Geometry: final body of the model. Coordinates: model frame, mm. Round coordinates to 2 decimals unless told otherwise and drop trailing zeros. Loops run counter-clockwise (first coordinate to the right, second up) from the corner with the lowest first, then second, coordinate; pieces in that order, holes last. Notation, with made-up numbers: M 21,11.5 L 67,11.5 A16 ccw 67,26.5 Z; hole C 31.25,6 d5. An arc over 180 degrees is marked long. Return JSON: item names as keys, results as strings.
from build123d import *

# Parameters (mm, degrees)
SKETCH1_R                    = 42.5
BOSS_EXTRUDE1_DEPTH          = 6
SKETCH2_R                    = 25.15
CUT_EXTRUDE1_DEPTH           = 61.402814504
SKETCH3_R                    = 2.25
CUT_EXTRUDE2_DEPTH           = 61.402814504
CHAMFER2_SIZE                = 2.2
CIRPATTERN1_COUNT            = 6
CHAMFER2_OF_CIRPATTERN1_SIZE = 2.2
CHAMFER1_SIZE                = 1
FILLET1_R                    = 1


with BuildPart() as part:
    # Sketch1 → Boss-Extrude1 (new body)
    with BuildSketch(Plane.XY):
        Circle(SKETCH1_R)
    extrude(amount=BOSS_EXTRUDE1_DEPTH)

    # Sketch2 → Cut-Extrude1 (cut, through all)
    with BuildSketch(Plane.XY.offset(6)):
        Circle(SKETCH2_R)
    extrude(amount=-CUT_EXTRUDE1_DEPTH, mode=Mode.SUBTRACT)

    # Sketch3 → Cut-Extrude2 (cut, through all)
    with BuildSketch(Plane.XY.offset(6)):
        with Locations((0, 35)):
            Circle(SKETCH3_R)
    cut_extrude2 = extrude(amount=-CUT_EXTRUDE2_DEPTH, mode=Mode.SUBTRACT)

    # Chamfer2
    chamfer2_edges = [part.edges().sort_by_distance(p)[0] for p in [
        (-2.25, 35, 6),
    ]]
    chamfer(chamfer2_edges, length=CHAMFER2_SIZE)

    # CirPattern1: Cut-Extrude2 ×6 about axis
    cirpattern1_axis = Axis((0, 0, 0), (0, 0, 1))
    for i in range(1, CIRPATTERN1_COUNT):
        add(cut_extrude2.rotate(cirpattern1_axis, i * 360 / CIRPATTERN1_COUNT), mode=Mode.SUBTRACT)

    # Chamfer2 of CirPattern1
    chamfer2_of_cirpattern1_edges = [part.edges().sort_by_distance(p)[0] for p in [
        (-31.435889132, 15.551442841, 6),
        (-29.185889132, -19.448557159, 6),
        (2.25, -35, 6),
        (31.435889132, -15.551442841, 6),
        (29.185889132, 19.448557159, 6),
    ]]
    chamfer(chamfer2_of_cirpattern1_edges, length=CHAMFER2_OF_CIRPATTERN1_SIZE)

    # Chamfer1
    chamfer1_edges = [part.edges().sort_by_distance(p)[0] for p in [
        (-25.15, 0, 0),
        (-25.15, 0, 6),
    ]]
    chamfer(chamfer1_edges, length=CHAMFER1_SIZE)

    # Fillet1
    fillet1_edges = [part.edges().sort_by_distance(p)[0] for p in [
        (-42.5, 0, 6),
    ]]
    fillet(fillet1_edges, radius=FILLET1_R)


solid = part.part
Q1. Section query A-A (y = 0). Output: boundary loops of the cut face in (x, z), plus the area to 3 significant figures.
Determined:
{"outline": "M -42.5,0 L -26.15,0 L -25.15,1 L -25.15,5 L -26.15,6 L -41.5,6 A1 ccw -42.5,5 Z; M 25.15,1 L 26.15,0 L 42.5,0 L 42.5,5 A1 ccw 41.5,6 L 26.15,6 L 25.15,5 Z", "area": "206 mm^2"}
Q2. Section query B-B (y = 17.5). State how many separate pieces and enclosed holes the cut face has, plus the area to 3 significant figures.
Determined:
{"separate pieces": "4", "enclosed holes": "0", "area": "181 mm^2"}
Q3. Pull-direction query (Y, two-part tool) for faces 1 (the conical face through (-28.06, -16.79, 3.91)), 2 (the cylindrical face through (-33.727, -25.861, 2.465)), 3 (the flat face through (18.3, 19.5, 0)); classes: pulls with the +Y half, pulls with the -Y half, needs draft (parallel to the pull), parting line crosses it, or undercut.
Determined:
{"face 1": "undercut", "face 2": "parting line crosses it", "face 3": "needs draft"}
Q4. Material intervals for L1, parallel to Y at x = 0, z = 2.05; L2, parallel to Y at x = 30, z = 2.5; L3, parallel to Y at x = -3.5, z = 5.4, sorted ascending.
Determined:
{"L1": "y = -42.5 to -37.25, -32.75 to -25.15, 25.15 to 32.75, 37.25 to 42.5", "L2": "y = -30.1 to -19.73, -15.27 to 15.27, 19.73 to 30.1", "L3": "y = -42.27 to -36.6, -33.4 to -25.31, 25.31 to 33.4, 36.6 to 42.27"}
Q5. Pin query (flat end, axial travel): pin 1 (3.5 mm diameter, centred on x = 30.31, y = 17.5, fed in from -Z); pin 2 (2 mm diameter, centred on x = 31.5, z = 5, fed in from +Y); pin 3 (2 mm diameter, centred on y = -19, z = 5, fed in from -X); pin 4 (3 mm diameter, centred on x = 17.5, z = 2.5, fed in from -Y). Return the tip coordinate at first contact, or that it passes through.
Determined:
{"pin 1": "passes through", "pin 2": "stops at y = 29.6", "pin 3": "stops at x = -38.5", "pin 4": "stops at y = -39.37"}
